Input: part model. Units: mm. Frame: model coordinates. Give positions to 0.01 mm unless a question says otherwise; leave off trailing zeros. Write each loop counter-clockwise with the first axis right and the second up, starting at its lowest first coordinate (ties: lowest second). Pieces come first, ordered by that corner, then holes. Notation, with made-up numbers: (68.25, -6) -> (103.25, -6) arc R28 cw to (103.25, 32) -> close; hole circle Ø6 at (-21.75, -6.75). An arc over 180 degrees is marked (long way). Answer as a JSON object with one key per item and string values. Group by question number.
Autodesk Inventor part; units mm, degrees
ref_plane "YZ Plane" through (0, 0, 0) normal (1, 0, 0) x (0, 1, 0)
ref_plane "XZ Plane" through (0, 0, 0) normal (0, 1, 0) x (-1, 0, 0)
ref_plane "XY Plane" through (0, 0, 0) normal (0, 0, 1) x (1, 0, 0)
sketch "Esboço1" plane through (0, 0, 0) normal (0, 0, 1) x (1, 0, 0)
  line L0 (-34.4331, 101.047) -> (41.7669, 101.047)
  line L1 (41.7669, 101.047) -> (41.7669, 91.027)
  line L2 (41.7669, 91.027) -> (-34.4331, 91.027)
  line L3 (-34.4331, 91.027) -> (-34.4331, 101.047)
  point P0 (0, 0)
  dimension "d0" = 76.2
  dimension "d1" = 10.02
extrude "Extrusão1" add sketch "Esboço1" along normal blind 30
sketch "Esboço2" plane through (-34.4331, 101.047, 0) normal (0, 1, 0) x (1, 0, 0)
  line L0 (76.2, 0) -> (76.2, -30)
  line L1 (76.2, -20) -> (0, -20)
  line L2 (0, 0) -> (0, -30)
  line L3 (0, 0) -> (76.2, 0)
  line L4 (38.1, -40) -> (38.1, 0)
  circle A0 centre (61.1, -20) radius 6.7139
  circle A1 centre (15.1, -20) radius 6.7459
  point P0 (34.4331, 0)
  dimension "d4" = 20
  dimension "d5" = 23
  dimension "d6" = 23
hole "Furo1" at (26.6669, 101.047, 20) at (-19.3331, 101.047, 20) direction (0, -1, 0) diameter 12.1 end through all
chamfer "Chanfro1" distance 2 angle 45 1 edges at (41.7669, 96.037, 30)
chamfer "Chanfro2" distance 2 angle 45 1 edges at (-34.4331, 96.037, 30)
equation "\"d6\" = d5"
equation "\"d12\" = 0.5 * d1"
properties part number "SuporteGuiasCabeçasAquecimentoUsinagem"
1. Mould query, pull axis X, two halves, no side actions, for faces 1 (the face through (4, 91.027, 15)), 2 (the face through (-17.02, 95.97, 25.59)), 3 (the face through (24.85, 95.97, 25.77)), 4 (the face through (-33.447, 95.967, 28.986)). Classes: pulls with the +X half, pulls with the -X half, needs draft (parallel to the pull), parting line crosses it, or undercut.
2. Section B-B (x = 25). Return the cut outline in (y, z).
3. Section A-A (z = 20). Return the cut outline in (x, y).
4. Line query: line 1 (X direction, y = 95.25, z = 20); line 2 (X direction, y = 100.5, z = 22.75); line 3 (Z direction, x = 24, y = 93.25). Output: solid intervals per line, ascending.
5. Section D-D (x = -23). Return the cut outline in (y, z), plus the area to 3 significant figures.
6. Section C-C (y = 93.75). Return the cut outline in (x, z), plus the area to 3 significant figures.
Working result:
{
 "1": {"face 1": "needs draft", "face 2": "undercut", "face 3": "undercut", "face 4": "pulls with the -X half"},
 "2": {"outline": "(91.03, 0) -> (101.05, 0) -> (101.05, 14.18) -> (91.03, 14.18) -> close; (91.03, 25.82) -> (101.05, 25.82) -> (101.05, 30) -> (91.03, 30) -> close"},
 "3": {"outline": "(-34.43, 91.03) -> (-25.38, 91.03) -> (-25.38, 101.05) -> (-34.43, 101.05) -> close; (-13.28, 91.03) -> (20.62, 91.03) -> (20.62, 101.05) -> (-13.28, 101.05) -> close; (32.72, 91.03) -> (41.77, 91.03) -> (41.77, 101.05) -> (32.72, 101.05) -> close"},
 "4": {"line 1": "x = -34.43 to -25.38, -13.28 to 20.62, 32.72 to 41.77", "line 2": "x = -34.43 to -24.72, -13.94 to 21.28, 32.06 to 41.77", "line 3": "z = 0 to 14.57, 25.43 to 30"},
 "5": {"outline": "(91.03, 0) -> (101.05, 0) -> (101.05, 15.19) -> (91.03, 15.19) -> close; (91.03, 24.81) -> (101.05, 24.81) -> (101.05, 30) -> (91.03, 30) -> close", "area": "204 mm^2"},
 "6": {"outline": "(-34.43, 0) -> (41.77, 0) -> (41.77, 28) -> (39.77, 30) -> (-32.43, 30) -> (-34.43, 28) -> close; hole circle Ø12.1 at (-19.33, 20); hole circle Ø12.1 at (26.67, 20)", "area": "2,050 mm^2"}
}
